Here's how the part is built. I have some questions about the finished solid (model axes, mm). A direction names the side the tool comes from. Round coordinates to 2 decimals unless told otherwise and drop trailing zeros. Order: outer loops, then holes, each group sorted by start corner. A loop starts at its lowest first (then second) coordinate and runs counter-clockwise, first axis right, second up. Notation, with made-up numbers: (-38, 22.25) -> (-7, 22.25) arc R17 ccw to (-7, 47.25) -> close; hole circle Ø10 at (36, 73.5). An arc over 180 degrees is marked (long way). One line per item, written item: value.
```python
from build123d import *

# Parameters (mm, degrees)
SKETCH1_W           = 267.5
SKETCH1_H           = 536
SKETCH1_R           = 2.75
BOSS_EXTRUDE1_DEPTH = 8
SKETCH3_R           = 2.75
SKETCH3_R_2         = 1.75
SKETCH3_R_3         = 3.5
SKETCH3_R_4         = 4
SKETCH3_R_5         = 3
SKETCH3_W           = 80
SKETCH3_H           = 53
CUT_EXTRUDE3_DEPTH  = 379.740346412
SKETCH4_R           = 1.75
SKETCH4_R_2         = 1.786950001
CUT_EXTRUDE4_DEPTH  = 10


with BuildPart() as part:
    # Sketch1 → Boss-Extrude1 (new body)
    with BuildSketch(Plane.XY):
        with Locations((133.75, 0)):
            Rectangle(SKETCH1_W, SKETCH1_H)
        with Locations(Location((257.5, -168, 0), (0, 0, 180))):
            Circle(SKETCH1_R, mode=Mode.SUBTRACT)
        with Locations(Location((257.509341423, -143.000001745, 0), (0, 0, 180))):
            Circle(SKETCH1_R, mode=Mode.SUBTRACT)
        with Locations((257.509341423, 143.000001745)):
            Circle(SKETCH1_R, mode=Mode.SUBTRACT)
        with Locations((257.5, 168)):
            Circle(SKETCH1_R, mode=Mode.SUBTRACT)
    extrude(amount=-BOSS_EXTRUDE1_DEPTH)

    # Sketch3 → Cut-Extrude3 (cut, through all)
    with BuildSketch(Plane.XY):
        with Locations(Location((257.509341423, -143.000001745, 0), (0, 0, 180))):
            Circle(SKETCH3_R)
        with Locations(Location((257.5, -168, 0), (0, 0, 180))):
            Circle(SKETCH3_R)
        with Locations((86.878100048, -154.208377346)):
            Circle(SKETCH3_R_2)
        with Locations((174.878100048, -154.208377346)):
            Circle(SKETCH3_R_2)
        with Locations((174.878100048, -219.208377346)):
            Circle(SKETCH3_R_2)
        with Locations((86.878100048, -219.208377346)):
            Circle(SKETCH3_R_2)
        with Locations((168.378100048, -230.458377346)):
            Circle(SKETCH3_R_3)
        with Locations((133.878100048, -230.708377346)):
            Circle(SKETCH3_R_4)
        with Locations((92.878100048, -227.708377346)):
            Circle(SKETCH3_R_5)
        with BuildLine():
            Line((0, 208), (0, -172))
            Line((0, -172), (31.225700951, -140.783627636))
            ThreePointArc((31.225700951, -140.783627636), (40.957302403, -134.282756532), (52.435734985, -132))
            Line((52.435734985, -132), (169.5, -132))
            ThreePointArc((169.5, -132), (190.713203436, -123.213203436), (199.5, -102))
            Line((199.5, -102), (199.5, 178))
            ThreePointArc((199.5, 178), (190.713203436, 199.213203436), (169.5, 208))
            Line((169.5, 208), (0, 208))
        make_face()
        Polygon((153.342201663, -229.708377346), (151.610150855, -226.708377346), (148.14604924, -226.708377346), (146.413998433, -229.708377346), (148.14604924, -232.708377346), (151.610150855, -232.708377346), align=None)
        with Locations((131.378100048, -186.208377346)):
            Rectangle(SKETCH3_W, SKETCH3_H)
    extrude(amount=-CUT_EXTRUDE3_DEPTH, mode=Mode.SUBTRACT)

    # Sketch4 → Cut-Extrude4 (cut)
    with BuildSketch(Plane.XY):
        with Locations((9.726391767, -172.881531455)):
            Circle(SKETCH4_R)
        with Locations((169.5, -139.5)):
            Circle(SKETCH4_R_2)
        with Locations((207, -102)):
            Circle(SKETCH4_R)
        with Locations((207, 38)):
            Circle(SKETCH4_R)
        with Locations((207, 178)):
            Circle(SKETCH4_R)
        with Locations((169.5, 215.5)):
            Circle(SKETCH4_R)
        with Locations((9.726391767, 215.5)):
            Circle(SKETCH4_R)
    extrude(amount=-CUT_EXTRUDE4_DEPTH, mode=Mode.SUBTRACT)


solid = part.part
```
Q1. I want a section at C-C on y = 69. Write out the boundary of the cut face in (x, z).
Answers:
outline: (199.5, -8) -> (267.5, -8) -> (267.5, 0) -> (199.5, 0) -> close
Q2. I want a section at A-A on x = 46.5. Write out the boundary of the cut face in (y, z).
Answers:
outline: (-268, -8) -> (-132.59, -8) -> (-132.59, 0) -> (-268, 0) -> close; (208, -8) -> (268, -8) -> (268, 0) -> (208, 0) -> close
Q3. I want a section at B-B on z = -5.25. Give the number of separate pieces and of enclosed holes in the cut face, then the cut area to 3 significant figures.
Answers:
separate pieces: 1
enclosed holes: 20
area: 70,500 mm2
Q4. If we mould it in two halves opening along Y, with no side actions, what happens to faces 3 (the face through (221, 4, -8)), 4 (the face through (190.479, -123.445, -3.944))? For each: pulls with the +Y half, pulls with the -Y half, needs draft (parallel to the pull), parting line crosses it, or undercut.
Answers:
face 3: needs draft
face 4: undercut
Q5. I need wall thicknesses on line 1 along Y through (x, z) = (207, -3.25); line 2 along X through (y, z) = (215.5, -2.75); line 3 along Y through (x, z) = (87, -6.25). Which ranges of each line are inside material? Lowest first, please.
Answers:
line 1: -268 to -103.75, -100.25 to 36.25, 39.75 to 176.25, 179.75 to 268
line 2: 0 to 7.98, 11.48 to 167.75, 171.25 to 267.5
line 3: -268 to -220.95, -217.46 to -155.95, -152.46 to -132, 208 to 268
Q6. Which directions (+Z, -Z, +X, -X, +Y, -Y) give clear straight access to the entire face, cutting with the end or side of a thin tool? Please do faces 1 (the face through (190.945, 198.979, -3.944)), 2 (the face through (221, 4, 0)).
Answers:
face 1: +Z, -Z, -X
face 2: +Z, +X, -X, +Y, -Y
